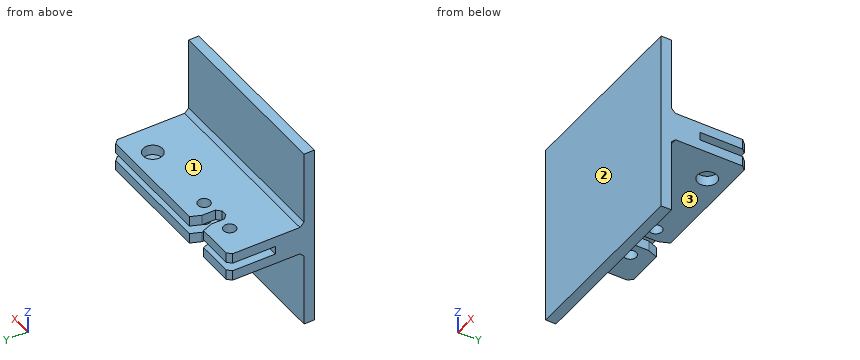
Autodesk Inventor part; units mm, degrees
ref_plane "YZ Plane" through (0, 0, 0) normal (1, 0, 0) x (0, 1, 0)
ref_plane "XZ Plane" through (0, 0, 0) normal (0, 1, 0) x (-1, 0, 0)
ref_plane "XY Plane" through (0, 0, 0) normal (0, 0, 1) x (1, 0, 0)
sketch "Sketch1" plane through (0, 0, 0) normal (0, 1, 0) x (-1, 0, 0)
  line L0 (0, 0) -> (90, 0)
  line L1 (90, 0) -> (90, -90)
  line L2 (90, -90) -> (0, -90)
  line L3 (0, -90) -> (0, 0)
  dimension "d0" = 90
  dimension "d1" = 90
extrude "Extrusion1" add sketch "Sketch1" along normal blind 5
sketch "Sketch2" plane through (0, 5, 0) normal (0, 1, 0) x (1, 0, 0)
  line L0 (-90, 90) -> (-90, 0) construction
  line L1 (-90, 45) -> (0, 45) construction
  line L2 (0, 0) -> (0, 90) construction
  line L3 (-90, 43) -> (0, 43)
  line L4 (0, 43) -> (0, 38)
  line L5 (0, 38) -> (-90, 38)
  line L6 (-90, 38) -> (-90, 43)
  line L7 (-90, 47) -> (0, 47)
  line L8 (0, 47) -> (0, 52)
  line L9 (0, 52) -> (-90, 52)
  line L10 (-90, 52) -> (-90, 47)
  dimension "d5" = 5
  dimension "d6" = 5
  dimension "d7" = 2
  dimension "d8" = 2
extrude "Extrusion2" add sketch "Sketch2" along normal blind 37
sketch "Sketch3" plane through (-90, 5, -38) normal (0, 0, 1) x (1, 0, 0)
  circle A0 centre (15, 27) radius 3
  circle A1 centre (35, 27) radius 3
  circle A2 centre (75, 27) radius 4.75
  line L0 (0, 0) -> (0, 37)
  line L1 (90, 0) -> (90, 37)
  line L2 (0, 37) -> (90, 37)
  line L3 (28.5, 25.5503) -> (26.4497, 23.5)
  line L4 (26.4497, 23.5) -> (23.5503, 23.5)
  line L5 (23.5503, 23.5) -> (21.5, 25.5503)
  line L6 (21.5, 25.5503) -> (28.5, 25.5503)
  point P0 (90, -5)
  point P1 (25, 27)
  point P2 (25, 27)
  dimension "d11" = 6
  dimension "d12" = 6
  dimension "d13" = 9.5
  dimension "d14" = 20
  dimension "d15" = 40
  dimension "d16" = 15
  dimension "d17" = 15
  dimension "d18" = 10
  dimension "d20" = 10
extrude "Extrusion3" cut sketch "Sketch3" against normal blind 14
sketch "Sketch4" plane through (-90, 5, -38) normal (0, 0, 1) x (1, 0, 0)
  line L0 (21.5, 25.5503) -> (28.5, 25.5503)
  line L1 (90, 37) -> (0, 37)
  line L2 (21.5, 25.5503) -> (28.5, 25.5503)
  line L3 (28.5, 25.5503) -> (28.5, 37)
  line L4 (28.5, 37) -> (21.5, 37)
  line L5 (21.5, 37) -> (21.5, 25.5503)
  point P0 (90, -5)
  dimension "d24" = 7
extrude "Extrusion4" cut sketch "Sketch4" against normal blind 14
sketch "Sketch5" plane through (0, 5, 0) normal (0, 1, 0) x (1, 0, 0)
  point P0 (0, 0)
sketch "Sketch6" plane through (0, 5, 0) normal (0, 1, 0) x (1, 0, 0)
  line L0 (-90, 47) -> (-90, 43)
  line L1 (0, 43) -> (0, 47)
  line L2 (-90, 43) -> (0, 43)
  line L3 (0, 43) -> (0, 47)
  line L4 (0, 47) -> (-90, 47)
  line L5 (-90, 47) -> (-90, 43)
  point P0 (0, 0)
extrude "Extrusion5" add sketch "Sketch6" along normal blind 14
chamfer "Chamfer1" distance 2 angle 45 6 edges at (-45, 5, -52) (0, 42, -40.5) (0, 42, -49.5) (-90, 42, -49.5) (-90, 42, -40.5) (-45, 5, -38)
chamfer "Chamfer2" distance 2 distance2 5 1 edges at (-68.5, 42, -40.5) measured on face at (-81.5, 42, -41.3333)
chamfer "Chamfer3" distance 2 distance2 5 1 edges at (-68.5, 42, -49.5) measured on face at (-81.5, 42, -50.3333)
chamfer "Chamfer4" distance 2 distance2 5 1 edges at (-61.5, 42, -49.5) measured on face at (-21.8333, 42, -48.6667)
chamfer "Chamfer5" distance 2 distance2 5 1 edges at (-61.5, 42, -40.5) measured on face at (-41.6667, 42, -41.3333)
The listing builds one solid part. Answer for the finished solid, in the listing's coordinates (mm). Face numbers are marked on the shaded views. A direction names the side the tool comes from. Give positions to 0.01 mm unless a question says otherwise; leave off trailing zeros. Write each loop counter-clockwise with the first axis right and the second up, starting at its lowest first coordinate (ties: lowest second). Pieces come first, ordered by that corner, then holes. Notation, with made-up numbers: (-12.75, 16.25) -> (25.25, 16.25) arc R23 cw to (25.25, 41.25) -> close; hole circle Ø9 at (19.25, 84.25). An arc over 180 degrees is marked (long way). Use one line per item in the form item = value.
1) Section A-A on x = -55 is taken. Write down the section's boundary in (y, z).
Result:
outline = (0, -90) -> (5, -90) -> (5, -54) -> (7, -52) -> (29, -52) -> (29, -47) -> (19, -47) -> (19, -43) -> (29, -43) -> (29, -38) -> (7, -38) -> (5, -36) -> (5, 0) -> (0, 0) -> close; (35, -52) -> (42, -52) -> (42, -47) -> (35, -47) -> close; (35, -43) -> (42, -43) -> (42, -38) -> (35, -38) -> close
2) Each of these flat-tipped pins is pushed along its axis until it touches: P1, Ø11, axis at x = -48, z = -69, coming from the +Y side; P2, Ø7, axis at x = -23, y = 34.5, coming from the +Z side; P3, Ø6, axis at x = -39, z = -34.5, coming from the +Y side. Where does it stop, or does it pass through?
Result:
P1 = 5
P2 = -38
P3 = 6.5
3) Straight lines are drawn through the part: probe 1 along Y at (x, z) = (-75, -39); probe 2 along Z at (x, y) = (-30, 30.5); probe 3 along Y at (x, z) = (-15, -39). For each, find the intervals that lie inside material, in ascending order.
Result:
probe_1 = 0 to 29, 35 to 42
probe_2 = -52 to -47, -43 to -38
probe_3 = 0 to 27.25, 36.75 to 42
4) Section C-C on x = -38 is taken. Write down the section's boundary in (y, z).
Result:
outline = (0, -90) -> (5, -90) -> (5, -54) -> (7, -52) -> (42, -52) -> (42, -47) -> (19, -47) -> (19, -43) -> (42, -43) -> (42, -38) -> (7, -38) -> (5, -36) -> (5, 0) -> (0, 0) -> close
5) A tool of negligible diameter and unlimited length cuts with its end or side. For the marked faces 1, 2 and 3, from which of +Z, -Z, +X, -X, +Y, -Y can it reach the whole face along a straight path? Write none if from no direction.
Result:
face_1 = +Z, +X, -X, +Y
face_2 = +Z, -Z, +X, -X, -Y
face_3 = -Z, +X, -X, +Y
6) Section D-D on z = -31 is taken. Write down the section's boundary in (x, y), plus the area to 3 significant figures.
Result:
outline = (-90, 0) -> (0, 0) -> (0, 5) -> (-90, 5) -> close
area = 450 mm²
7) Section B-B on y = 25.5 is taken. Write down the section's boundary in (x, z), plus the area to 3 significant figures.
Result:
outline = (-90, -52) -> (0, -52) -> (0, -47) -> (-90, -47) -> close; (-90, -43) -> (0, -43) -> (0, -38) -> (-90, -38) -> close
area = 900 mm²
